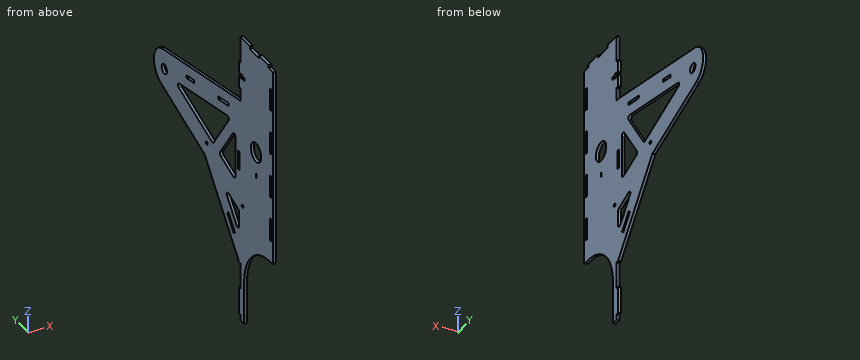
from build123d import *

# Parameters (mm, degrees)
BOSS_EXTRUDE1_DEPTH     = 3
SKETCH2_W               = 27.727272727
SKETCH2_H               = 3
SKETCH2_W_2             = 3
SKETCH2_H_2             = 18
SKETCH2_H_3             = 9
SKETCH2_W_3             = 23.343342349
SKETCH2_W_4             = 23.34334235
SKETCH2_W_5             = 6
CUT_EXTRUDE1_DEPTH      = 1
CUT_EXTRUDE1_DEPTH_BACK = 4
SKETCH3_W               = 3.2
SKETCH3_H               = 10.5
SKETCH3_W_2             = 5.2
SKETCH3_H_2             = 2.5
CUT_EXTRUDE2_DEPTH      = 1
CUT_EXTRUDE2_DEPTH_BACK = 4
FILLET1_R               = 2.5
BOSS_EXTRUDE2_DEPTH     = 3
FILLET2_R               = 2.5
SKETCH6_R               = 5
SKETCH6_R_2             = 1.65
CUT_EXTRUDE5_DEPTH      = 1
CUT_EXTRUDE5_DEPTH_BACK = 4
SKETCH8_R               = 10
SKETCH8_W               = 5
SKETCH8_H               = 1
CUT_EXTRUDE6_DEPTH      = 4
CUT_EXTRUDE6_DEPTH_BACK = 1
SKETCH9_W               = 20
SKETCH9_H               = 3
CUT_EXTRUDE7_DEPTH      = 4
CUT_EXTRUDE7_DEPTH_BACK = 1
SKETCH10_W              = 27.840909091
SKETCH10_H              = 3
CUT_EXTRUDE8_DEPTH      = 4
CUT_EXTRUDE8_DEPTH_BACK = 1


with BuildPart() as part:
    # Sketch1 → Boss-Extrude1 (new body)
    with BuildSketch(Plane(origin=(0, 0, 0), x_dir=(0, 0, -1), z_dir=(1, 0, 0))):
        with BuildLine():
            Line((-152.5, 33), (152.5, 33))
            Line((152.5, 33), (152.5, 23))
            Line((152.5, 23), (107.5, 23))
            ThreePointArc((107.5, 23), (72.144660941, 8.355339059), (57.5, -27))
            Line((57.5, -27), (57.5, -33))
            Line((57.5, -33), (-152.5, -33))
            Line((-152.5, -33), (-152.5, 33))
        make_face()
    extrude(amount=BOSS_EXTRUDE1_DEPTH)

    # Sketch2 → Cut-Extrude1 (cut, two sides)
    with BuildSketch(Plane(origin=(3, 0, 0), x_dir=(0, 0, -1), z_dir=(1, 0, 0))) as cut_extrude1_sk:
        with Locations((-138.636363636, 31.5)):
            Rectangle(SKETCH2_W, SKETCH2_H)
        with Locations((-83.181818182, 31.5)):
            Rectangle(SKETCH2_W, SKETCH2_H)
        with Locations((-27.727272728, 31.5)):
            Rectangle(SKETCH2_W, SKETCH2_H)
        with Locations((-151, 3)):
            Rectangle(SKETCH2_W_2, SKETCH2_H_2)
        with Locations((-151, -28.5)):
            Rectangle(SKETCH2_W_2, SKETCH2_H_3)
        with Locations((-117.484986475, -28.5)):
            Rectangle(SKETCH2_W_3, SKETCH2_H)
        with Locations((-70.798301777, -28.5)):
            Rectangle(SKETCH2_W_3, SKETCH2_H)
        with Locations((22.575067622, -28.5)):
            Rectangle(SKETCH2_W_4, SKETCH2_H)
        with Locations((149.5, 31.5)):
            Rectangle(SKETCH2_W_5, SKETCH2_H)
        with Locations((-24.111617078, -28.5)):
            Rectangle(SKETCH2_W_3, SKETCH2_H)
    extrude(amount=CUT_EXTRUDE1_DEPTH, mode=Mode.SUBTRACT)
    extrude(cut_extrude1_sk.sketch, amount=-CUT_EXTRUDE1_DEPTH_BACK, mode=Mode.SUBTRACT)

    # Sketch3 → Cut-Extrude2 (cut, two sides)
    with BuildSketch(Plane(origin=(3, 0, 0), x_dir=(0, 0, -1), z_dir=(1, 0, 0))) as cut_extrude2_sk:
        with Locations((-110.909090909, 27.75)):
            Rectangle(SKETCH3_W, SKETCH3_H)
        with Locations((-110.909090909, 28.575)):
            Rectangle(SKETCH3_W_2, SKETCH3_H_2)
    extrude(amount=CUT_EXTRUDE2_DEPTH, mode=Mode.SUBTRACT)
    extrude(cut_extrude2_sk.sketch, amount=-CUT_EXTRUDE2_DEPTH_BACK, mode=Mode.SUBTRACT)

    # Fillet1
    fillet1_edges = [part.edges().sort_by_distance(p)[0] for p in [
        (1.5, -33, -57.5),
    ]]
    fillet(fillet1_edges, radius=FILLET1_R)

    # Sketch4 → Boss-Extrude2 (add)
    with BuildSketch(Plane(origin=(0, 0, 0), x_dir=(0, 0, -1), z_dir=(1, 0, 0))):
        with BuildLine():
            Line((-83.181818182, 33), (-83.181818182, 30))
            Line((-83.181818182, 30), (35.818181818, 30))
            Line((35.818181818, 30), (35.818181818, 33))
            Line((35.818181818, 33), (25.753026775, 61.931534749))
            Line((25.753026775, 61.931534749), (59.886459158, 33))
            Line((59.886459158, 33), (90.818181818, 33))
            Line((90.818181818, 33), (12.817635516, 99.113348651))
            Line((12.817635516, 99.113348651), (-16.565017269, 183.571584658))
            ThreePointArc((-16.565017269, 183.571584658), (-36.922973482, 196.946020133), (-55.102803407, 180.73442893))
            Line((-55.102803407, 180.73442893), (-83.181818182, 33))
        make_face()
        Polygon((-54.643252411, 49.263022537), (-34.033564648, 157.698467174), (-8.047004759, 83.002045982), align=None, mode=Mode.SUBTRACT)
        Polygon((-3.929894771, 71.167721507), (6.913219914, 40), (-46.974972009, 40), align=None, mode=Mode.SUBTRACT)
    extrude(amount=BOSS_EXTRUDE2_DEPTH)

    # Fillet2
    fillet2_edges = [part.edges().sort_by_distance(p)[0] for p in [
        (1.5, 33, -59.886459158),
        (1.5, 61.931534749, -25.753026775),
        (1.5, 33, -35.818181818),
        (1.5, 40, -6.913219914),
        (1.5, 71.167721507, 3.929894771),
        (1.5, 40, 46.974972009),
        (1.5, 49.263022537, 54.643252411),
        (1.5, 83.002045982, 8.047004759),
        (1.5, 157.698467174, 34.033564648),
    ]]
    fillet(fillet2_edges, radius=FILLET2_R)

    # Sketch6 → Cut-Extrude5 (cut, two sides)
    with BuildSketch(Plane(origin=(3, 0, 0), x_dir=(0, 0, -1), z_dir=(1, 0, 0))) as cut_extrude5_sk:
        with Locations((-35.454545455, 177)):
            Circle(SKETCH6_R)
        with Locations((-1.492946709, 95.333591431)):
            Circle(SKETCH6_R_2)
        with Locations((27.342535354, 25.993797473)):
            Circle(SKETCH6_R_2)
    extrude(amount=CUT_EXTRUDE5_DEPTH, mode=Mode.SUBTRACT)
    extrude(cut_extrude5_sk.sketch, amount=-CUT_EXTRUDE5_DEPTH_BACK, mode=Mode.SUBTRACT)

    # Sketch8 → Cut-Extrude6 (cut, two sides)
    with BuildSketch(Plane(origin=(0, 0, 0), x_dir=(0, 0, -1), z_dir=(1, 0, 0))) as cut_extrude6_sk:
        with Locations((-45, 0)):
            Circle(SKETCH8_R)
        with Locations((-20, 0)):
            Rectangle(SKETCH8_W, SKETCH8_H)
    extrude(amount=CUT_EXTRUDE6_DEPTH, mode=Mode.SUBTRACT)
    extrude(cut_extrude6_sk.sketch, amount=-CUT_EXTRUDE6_DEPTH_BACK, mode=Mode.SUBTRACT)

    # Sketch9 → Cut-Extrude7 (cut, two sides)
    with BuildSketch(Plane(origin=(0, 0, 0), x_dir=(0, 0, -1), z_dir=(1, 0, 0))) as cut_extrude7_sk:
        Polygon((-68.111670983, 53.378521315), (-64.377242053, 73.026779267), (-61.43000336, 72.466614928), (-65.16443229, 52.818356975), align=None)
        Polygon((-55.507973344, 119.691391905), (-52.707151647, 134.427585369), (-49.759912954, 133.867421029), (-52.560734651, 119.131227565), align=None)
        Polygon((64.311409407, 40.391956194), (49.054577079, 53.32366402), (50.994333253, 55.612188869), (66.251165581, 42.680481043), align=None)
        with Locations((-17.931502251, 33)):
            Rectangle(SKETCH9_W, SKETCH9_H)
    extrude(amount=CUT_EXTRUDE7_DEPTH, mode=Mode.SUBTRACT)
    extrude(cut_extrude7_sk.sketch, amount=-CUT_EXTRUDE7_DEPTH_BACK, mode=Mode.SUBTRACT)

    # Sketch10 → Cut-Extrude8 (cut, two sides)
    with BuildSketch(Plane(origin=(0, 0, 0), x_dir=(0, 0, -1), z_dir=(1, 0, 0))) as cut_extrude8_sk:
        with Locations((104.738636364, 31.5)):
            Rectangle(SKETCH10_W, SKETCH10_H)
    extrude(amount=CUT_EXTRUDE8_DEPTH, mode=Mode.SUBTRACT)
    extrude(cut_extrude8_sk.sketch, amount=-CUT_EXTRUDE8_DEPTH_BACK, mode=Mode.SUBTRACT)


solid = part.part
The model under review builds one solid part; all positions refer to its coordinate system, in mm. Round coordinates to 2 decimals unless told otherwise and drop trailing zeros. Order: outer loops, then holes, each group sorted by start corner. A loop starts at its lowest first (then second) coordinate and runs counter-clockwise, first axis right, second up. Notation, with made-up numbers: (-38.75, 71.25) -> (-6.75, 71.25) arc R9 ccw to (-6.75, 80.25) -> close; hole circle Ø9 at (-30, 58.25). An arc over 180 degrees is marked (long way). Use CSV: the item, a comma, the result in double quotes. Start each with the question number.
(1) Consider section C-C on z = 101. Write out the cut boundary in (x, y).
(2) Insertion check: pin 1 (0.9 mm diameter, centred on x = 2, z = 119.5, fed in from +Y); pin 2 (1.5 mm diameter, centred on x = 1, z = 28.5, fed in from +Y); pin 3 (1.5 mm diameter, centred on x = 1.5, y = -29, fed in from -Z). Each pin has a flat end and moves straight along its axis. Give the tip position at first contact, or say it passes through.
(3) Consider section B-B on z = 45. Write out the cut boundary in (x, y), and give its area (3 significant figures).
(4) Consider section A-A on y = 177. Write out the cut boundary in (x, z), and give its area (3 significant figures).
(5) Consider section D-D on x = 0.75. State how many separate pieces and enclosed holes the cut face has, and give its area (3 significant figures).
(6) Wall thickness on probe 1 along Y at (x, z) = (1.6, 121); probe 2 along Z at (x, y) = (0.4, 43.5); probe 3 along Z at (x, y) = (2.2, 63.5): over which ranges is each line inside the solid? List them lowest first. Write a range as from..to.
Responses:
1,outline,"(0, -33) -> (3, -33) -> (3, 33) -> (0, 33) -> close"
2,pin 1,"y = 33"
2,pin 2,"y = 196.01"
2,pin 3,"z = -57.5"
3,outline,"(0, -33) -> (3, -33) -> (3, -10) -> (0, -10) -> close; (0, 10) -> (3, 10) -> (3, 56.25) -> (0, 56.25) -> close; (0, 100) -> (3, 100) -> (3, 194.58) -> (0, 194.58) -> close"
3,area,"491 mm²"
4,outline,"(0, 14.28) -> (3, 14.28) -> (3, 30.45) -> (0, 30.45) -> close; (0, 40.45) -> (3, 40.45) -> (3, 55.81) -> (0, 55.81) -> close"
4,area,"94.6 mm²"
5,separate pieces,"1"
5,enclosed holes,"16"
5,area,"24,800 mm²"
6,probe 1,"-33..-30, -27..33"
6,probe 2,"-78.43..-65.28, -60.64..-47.5, -32.17..-5.7, 41.55..81.19"
6,probe 3,"-54.83..1.26, 14.52..34.98, 51.94..63.13, 66.19..77.38"
